Autodesk Inventor part; units mm, degrees
ref_plane "YZ Plane" through (0, 0, 0) normal (1, 0, 0) x (0, 1, 0)
ref_plane "XZ Plane" through (0, 0, 0) normal (0, 1, 0) x (-1, 0, 0)
ref_plane "XY Plane" through (0, 0, 0) normal (0, 0, 1) x (1, 0, 0)
sketch "Sketch1" plane through (0, 0, 0) normal (0, 1, 0) x (-1, 0, 0)
  line L0 (0, 0) -> (0, 182) construction
  line L1 (0, 182) -> (46.8, 182) construction
  line L2 (46.8, 182) -> (46.8, 91)
  line L3 (46.8, 91) -> (55, 91)
  line L4 (55, 91) -> (55, 0)
  line L5 (55, 0) -> (63.2, 0)
  line L6 (63.2, 0) -> (63.2, 182)
  line L7 (63.2, 182) -> (46.8, 182)
  line L8 (55, 0) -> (0, 0) construction
  line L9 (0, 182) -> (0, 385) construction
  line L10 (0, 385) -> (-143.5427, 528.5427) construction
  line L11 (-143.5427, 528.5427) -> (-110.4501, 561.6353) construction
  line L12 (-110.4501, 561.6353) -> (-174.535, 625.7202)
  line L13 (-174.535, 625.7202) -> (-168.7367, 631.5185)
  line L14 (-168.7367, 631.5185) -> (-233.3452, 696.127)
  line L15 (-233.3452, 696.127) -> (-227.547, 701.9253)
  line L16 (-227.547, 701.9253) -> (-98.8535, 573.2318)
  line L17 (-110.4501, 561.6353) -> (-98.8535, 573.2318)
  line L18 (-143.5427, 528.5427) -> (-272.2361, 657.2361) construction
  line L19 (-233.3452, 696.127) -> (-272.2361, 657.2361) construction
  line L20 (0, 182) -> (-490.0854, 182) construction
  line L21 (-143.5427, 528.5427) -> (-490.0854, 182) construction
  arc A0 (0, 182) -> (-143.5427, 528.5427) centre (-490.0854, 182) ccw
  line L22 (-143.5427, 528.5427) -> (-143.5427, 182) construction
  line L23 (46.8, 91) -> (0, 91) construction
  line L24 (-174.535, 625.7202) -> (-207.6276, 592.6276) construction
  dimension "d0" = 182
  dimension "d1" = 91
  dimension "d2" = 93.6
  dimension "d3" = 110
  dimension "d4" = 126.4
  dimension "d5" = 203
  dimension "d6" = 203
  dimension "d7" = 182
  dimension "d8" = 91
  dimension "d9" = 93.6
  dimension "d10" = 110
  dimension "d11" = 126.4
  dimension "d12" = 45
revolve "Revolve1" add sketch "Sketch1" angle 360 about axis through (0, 0, 0) along (0, 0, 1) contours L7 L6 L5 L4 L3 L2
revolve "Revolve2" add sketch "Sketch1" angle 360 about axis through (143.5427, 0, 528.5427) along (0.7071068, 0, 0.7071068) contours L12 L13 L14 L15 L16 L17
sketch "Sketch2" plane through (0, 0, 182) normal (0, 0, 1) x (1, 0, 0)
  circle A0 centre (0, 0) radius 46.8
  circle A1 centre (0, 0) radius 55
sweep "Sweep1" add profiles "Sketch2" path "Sketch1" path curves A0
equation "\"d0\" = 2 * tk"
equation "\"d1\" = tk"
equation "\"d2\" = d - 2 * s1"
equation "\"d3\" = d"
equation "\"d4\" = d + 2 * s1"
equation "\"d5\" = zk"
equation "\"d6\" = zk"
equation "\"d7\" = 2 * tk"
equation "\"d8\" = tk"
equation "\"d9\" = d - 2 * s1"
equation "\"d10\" = d"
equation "\"d11\" = d + 2 * s1"
equation "\"zk\" = 203"
equation "\"tk\" = 91"
equation "\"d\" = 110"
equation "\"s1\" = 8.2"
properties part number "DIN 8063 Двойная подвижная соединительная муфта с изгибом 45 градусов со стыковой сваркой - MMK - KK 110 - 5" material "ПВХ, непластифицированный"
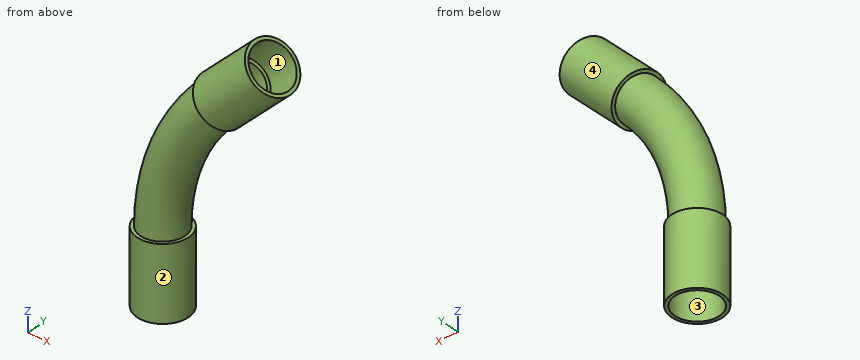
Build history of the part. All positions in model axes, mm. Face numbers are marked on the shaded views. A direction names the side the tool comes from. Coordinates: 2 decimals unless noted, no trailing zeros. Order: outer loops, then holes, each group sorted by start corner. A loop starts at its lowest first (then second) coordinate and runs counter-clockwise, first axis right, second up. Notation, with made-up numbers: (56, 9) -> (71, 9) arc R21 ccw to (71, 20) -> close; hole circle Ø2 at (45.25, 68). An arc over 180 degrees is marked (long way). Answer in a Markdown table with one row per item. Add a question column.
Q1. Drop flat-ended pins along their axis: pin 1 (12 mm diameter, centred on x = 216.5, z = 511, fed in from -Y); pin 2 (1 mm diameter, centred on x = 229, y = 50, fed in from -Z); pin 3 (8 mm diameter, centred on x = 187, y = 5, fed in from +Z). Give the stop position or say it passes through.
Q2. Band-saw the part on A-A, the plane z = 128.5. List the corners of the cut face in (x, y), then the cut area to 3 significant figures.
Q3. Wall check: line 1 along Y through (x, z) = (0, 22); line 2 along X through (y, z) = (0, 137). Give the ranges that are in metal, low to high. Write a range as [from, to].
Q4. Which spindle directions (+Z, -Z, +X, -X, +Y, -Y) get a long thin tool onto all of the face, cutting with end or side? Do the marked faces 1 and 2. Say none if no direction does.
Q5. Mould opens along Y. For the marked faces 3 and 4 say: +Y half, -Y half, draft (parallel to the pull), parting line (faces both ways), or undercut.
Q6. Band-saw the part on B-B, the plane z = 52.5. List the corners of the cut face in (x, y), then the cut area to 3 significant figures.
Answers follow:
| question | item | result |
|---|---|---|
| 1 | pin 1 | y = -25.12 |
| 1 | pin 2 | z = 558.3 |
| 1 | pin 3 | z = 665.12 |
| 2 | outline | circle Ø126.4 at (0, 0); hole circle Ø93.6 at (0, 0) |
| 2 | area | 5,670 mm^2 |
| 3 | line 1 | [-63.2, -55], [55, 63.2] |
| 3 | line 2 | [-63.2, -46.8], [46.8, 63.2] |
| 4 | face 1 | none |
| 4 | face 2 | -Z |
| 5 | face 3 | undercut |
| 5 | face 4 | parting line |
| 6 | outline | circle Ø126.4 at (0, 0); hole circle Ø110 at (0, 0) |
| 6 | area | 3,040 mm^2 |
